```python
from build123d import *

# Parameters (mm, degrees)
SKETCH_W        = 32
SKETCH_H        = 95
PAD_DEPTH       = 77
SKETCH001_W     = 29
SKETCH001_H     = 92
POCKET_DEPTH    = 77.001
SKETCH002_W     = 11
SKETCH002_H     = 1.5
SKETCH002_W_2   = 29
SKETCH002_H_2   = 30
SKETCH002_H_3   = 13
POCKET001_DEPTH = 95.001
SKETCH003_R     = 1.25
SKETCH003_R_2   = 1.5
SKETCH003_R_3   = 11
POCKET002_DEPTH = 32.001
SKETCH004_R     = 1.5
POCKET003_DEPTH = 32.001


with BuildPart() as part:
    # Sketch → Pad (new body)
    with BuildSketch(Plane.XZ):
        with Locations((-16, 47.5)):
            Rectangle(SKETCH_W, SKETCH_H)
    extrude(amount=PAD_DEPTH)

    # Sketch001 (on Face5 of Pad) → Pocket (cut, through all)
    with BuildSketch(Plane(origin=(0, 0, 0), x_dir=(1, 0, 0), z_dir=(0, 1, 0))):
        with Locations((-17.5, -49)):
            Rectangle(SKETCH001_W, SKETCH001_H)
    extrude(amount=-POCKET_DEPTH, mode=Mode.SUBTRACT)

    # Sketch002 (on Face1 of Pocket) → Pocket001 (cut, through all)
    with BuildSketch(Plane(origin=(0, 0, 0), x_dir=(1, 0, 0), z_dir=(0, 0, -1))):
        with Locations((-26.5, 11.25)):
            Rectangle(SKETCH002_W, SKETCH002_H)
        with Locations((-26.5, 5.75)):
            Rectangle(SKETCH002_W, SKETCH002_H)
        with Locations((-26.5, 58.25)):
            Rectangle(SKETCH002_W, SKETCH002_H)
        with Locations((-26.5, 52.75)):
            Rectangle(SKETCH002_W, SKETCH002_H)
        with Locations((-17.5, 32)):
            Rectangle(SKETCH002_W_2, SKETCH002_H_2)
        with Locations((-17.5, 70.5)):
            Rectangle(SKETCH002_W_2, SKETCH002_H_3)
    extrude(amount=-POCKET001_DEPTH, mode=Mode.SUBTRACT)

    # Sketch003 (on Face27 of Pocket001) → Pocket002 (cut, through all)
    with BuildSketch(Plane(origin=(0, 0, 0), x_dir=(0, 0, 1), z_dir=(1, 0, 0))):
        with Locations((20, 37.5)):
            Circle(SKETCH003_R)
        with Locations((20, 24)):
            Circle(SKETCH003_R)
        with Locations((47.5, 49)):
            Circle(SKETCH003_R)
        with Locations((47.5, 14)):
            Circle(SKETCH003_R)
        with Locations((59, 57)):
            Circle(SKETCH003_R_2)
        with Locations((90, 57)):
            Circle(SKETCH003_R_2)
        with Locations((90, 26)):
            Circle(SKETCH003_R_2)
        with Locations((59, 26)):
            Circle(SKETCH003_R_2)
        with Locations((74.5, 41.5)):
            Circle(SKETCH003_R_3)
        with Locations((75, 5)):
            Circle(SKETCH003_R)
        with Locations((91, 5)):
            Circle(SKETCH003_R)
        with Locations((31.5, 68.5)):
            Circle(SKETCH003_R)
        with Locations((41, 68.5)):
            Circle(SKETCH003_R)
    extrude(amount=-POCKET002_DEPTH, mode=Mode.SUBTRACT)

    # Sketch004 (on Face27 of Pocket002) → Pocket003 (cut, through all)
    with BuildSketch(Plane(origin=(0, 0, 0), x_dir=(0, 0, 1), z_dir=(1, 0, 0))):
        with Locations((6.5, 30)):
            Circle(SKETCH004_R)
        with Locations((26.5, 30)):
            Circle(SKETCH004_R)
        with Locations((26.5, 45)):
            Circle(SKETCH004_R)
        with Locations((6.5, 45)):
            Circle(SKETCH004_R)
    extrude(amount=-POCKET003_DEPTH, mode=Mode.SUBTRACT)


solid = part.part
```
For this review, take the finished solid that the model builds, in its own axes (mm). A direction names the side the tool comes from. Coordinates: 2 decimals unless noted, no trailing zeros. Loops run counter-clockwise (first coordinate to the right, second up) from the corner with the lowest first, then second, coordinate; pieces in that order, holes last. Notation, with made-up numbers: (70, -38.5) -> (85, -38.5) arc R5 ccw to (85, -31.5) -> close; hole circle Ø8 at (72.25, -3.5). An arc over 180 degrees is marked (long way). Return JSON: item names as keys, results as strings. Group by question number.
(1) To check wall thickness, follow L1, parallel to Z at x = -1, y = -26; L2, parallel to Y at x = -1.2, z = 6.5; L3, parallel to Z at x = -2.3, y = -41.5. State the ranges of each line that lie inside material, in increasing order.
(2) Consider section D-D, the plane x = -24. Give the boundary of the cut face in (y, z).
(3) Tool access review of faces 4 (the flat face through (-18, -17, 1)), 5 (the flat face through (-32, -55, 1)), 6 (the flat face through (-18, -64, 1)): name each direction out of +Z, -Z, +X, -X, +Y, -Y from which nothing blocks a thin tool from reaching the whole face with its end or side.
(4) For pin 1 Ø12 at (x, z) = (-6, 35) entering from +Y; pin 2 Ø3.5 at (y, z) = (-30, 6.5) entering from -X; pin 3 Ø2.5 at (x, z) = (-26.5, 1) entering from -Y; pin 4 Ø5 at (x, y) = (-17, -52.5) entering from +Z, all flat-tipped, find the tip position at first contact; note any pin that passes through.
(5) Consider section A-A, the plane z = 6.5. Give the boundary of the cut face in (x, y).
(6) Consider section B-B, the plane x = -8.5. Give the boundary of the cut face in (y, z).
(7) Consider section C-C, the plane y = -49. Give the boundary of the cut face in (x, z), plus the area to 3 significant figures.
(8) Mouldability with a two-part tool opening along Z and no side actions: class faces 1 (the cylindrical face through (-1.48, -69.74, 40.84)), 2 (the flat face through (-18, -8, 3)), 3 (the flat face through (-32, -14, 1)) as pulls with the +Z half, pulls with the -Z half, needs draft (parallel to the pull), parting line crosses it, or undercut.
Results below:
{
 "1": {"L1": "z = 0 to 57.5, 60.5 to 88.5, 91.5 to 95", "L2": "y = -77 to -46.5, -43.5 to -31.5, -28.5 to 0", "L3": "z = 0 to 63.5, 85.5 to 95"},
 "2": {"outline": "(-64, 0) -> (-59, 0) -> (-59, 3) -> (-64, 3) -> close; (-57.5, 0) -> (-53.5, 0) -> (-53.5, 3) -> (-57.5, 3) -> close; (-52, 0) -> (-47, 0) -> (-47, 3) -> (-52, 3) -> close; (-17, 0) -> (-12, 0) -> (-12, 3) -> (-17, 3) -> close; (-10.5, 0) -> (-6.5, 0) -> (-6.5, 3) -> (-10.5, 3) -> close; (-5, 0) -> (0, 0) -> (0, 3) -> (-5, 3) -> close"},
 "3": {"face 4": "+Z, -Z, -X", "face 5": "+Z, -Z, -X, +Y, -Y", "face 6": "+Z, -Z, -X, -Y"},
 "4": {"pin 1": "stops at y = 0", "pin 2": "stops at x = -3", "pin 3": "stops at y = -64", "pin 4": "stops at z = 3"},
 "5": {"outline": "(-3, -77) -> (0, -77) -> (0, -46.5) -> (-3, -46.5) -> close; (-3, -43.5) -> (0, -43.5) -> (0, -31.5) -> (-3, -31.5) -> close; (-3, -28.5) -> (0, -28.5) -> (0, 0) -> (-3, 0) -> close"},
 "6": {"outline": "(-64, 0) -> (-47, 0) -> (-47, 3) -> (-64, 3) -> close; (-17, 0) -> (0, 0) -> (0, 3) -> (-17, 3) -> close"},
 "7": {"outline": "(-32, 0) -> (0, 0) -> (0, 46.25) -> (-3, 46.25) -> (-3, 3) -> (-32, 3) -> close; (-3, 48.75) -> (0, 48.75) -> (0, 66.45) -> (-3, 66.45) -> close; (-3, 82.55) -> (0, 82.55) -> (0, 95) -> (-3, 95) -> close", "area": "316 mm2"},
 "8": {"face 1": "undercut", "face 2": "pulls with the +Z half", "face 3": "needs draft"}
}
